from build123d import *

# Parameters (mm, degrees)
ESBO_O1_R                                      = 4.7625
RESSALTO_EXTRUS_O1_DEPTH                       = 151.9
FURO_ROSCADO_DE_M5X0_81_D                      = 4.2
FURO_ROSCADO_DE_M5X0_81_DEPTH                  = 14
FURO_ROSCADO_DE_M5X0_81_TIP                    = 1.2618073
FILETE1_R                                      = 0.5
BROCA_DE_ROSQUEAR_PARA_TARRAXA_DE_M3X0_5_D     = 2.5
BROCA_DE_ROSQUEAR_PARA_TARRAXA_DE_M3X0_5_DEPTH = 5
BROCA_DE_ROSQUEAR_PARA_TARRAXA_DE_M3X0_5_TIP   = 0.751075774
FILETE2_R                                      = 0.5
BROCA_DE_ROSQUEAR_PARA_TARRAXA_DE_M3_2_D       = 2.5
BROCA_DE_ROSQUEAR_PARA_TARRAXA_DE_M3_2_DEPTH   = 10
BROCA_DE_ROSQUEAR_PARA_TARRAXA_DE_M3_2_TIP     = 0.751075774


with BuildPart() as part:
    # Esboço1 → Ressalto-extrusão1 (new body)
    with BuildSketch(Plane.XY):
        with Locations((21.9, 0.462441068)):
            Circle(ESBO_O1_R)
    extrude(amount=RESSALTO_EXTRUS_O1_DEPTH)

    # Furo roscado de M5x0.81
    with Locations(Plane(origin=(0, 0, 0), x_dir=(-1, 0, 0), z_dir=(0, 0, -1))):
        with Locations((-21.9, 0.462441068)):
            Hole(FURO_ROSCADO_DE_M5X0_81_D / 2, depth=FURO_ROSCADO_DE_M5X0_81_DEPTH)
            with Locations((0, 0, -(FURO_ROSCADO_DE_M5X0_81_DEPTH + FURO_ROSCADO_DE_M5X0_81_TIP / 2))):  # 118° drill point
                Cone(0, FURO_ROSCADO_DE_M5X0_81_D / 2, FURO_ROSCADO_DE_M5X0_81_TIP, mode=Mode.SUBTRACT)

    # Filete1
    filete1_edges = [part.edges().sort_by_distance(p)[0] for p in [
        (17.1375, 0.462441068, 0),
    ]]
    fillet(filete1_edges, radius=FILETE1_R)

    # Broca de rosquear para tarraxa de M3x0.5
    with Locations(Plane.XY.offset(151.9)):
        with Locations((21.9, 0.462441068)):
            Hole(BROCA_DE_ROSQUEAR_PARA_TARRAXA_DE_M3X0_5_D / 2, depth=BROCA_DE_ROSQUEAR_PARA_TARRAXA_DE_M3X0_5_DEPTH)
            with Locations((0, 0, -(BROCA_DE_ROSQUEAR_PARA_TARRAXA_DE_M3X0_5_DEPTH + BROCA_DE_ROSQUEAR_PARA_TARRAXA_DE_M3X0_5_TIP / 2))):  # 118° drill point
                Cone(0, BROCA_DE_ROSQUEAR_PARA_TARRAXA_DE_M3X0_5_D / 2, BROCA_DE_ROSQUEAR_PARA_TARRAXA_DE_M3X0_5_TIP, mode=Mode.SUBTRACT)

    # Filete2
    filete2_edges = [part.edges().sort_by_distance(p)[0] for p in [
        (17.1375, 0.462441068, 151.9),
    ]]
    fillet(filete2_edges, radius=FILETE2_R)

    # Broca de rosquear para tarraxa de M3 2
    with Locations(Plane(origin=(18.970347391, -3.292361436, 26.879843119), x_dir=(-0.78840997447, 0.615150154154, 0), z_dir=(-0.615150154154, -0.78840997447, 0))):
        with Locations((0, 0)):
            Hole(BROCA_DE_ROSQUEAR_PARA_TARRAXA_DE_M3_2_D / 2, depth=BROCA_DE_ROSQUEAR_PARA_TARRAXA_DE_M3_2_DEPTH)
            with Locations((0, 0, -(BROCA_DE_ROSQUEAR_PARA_TARRAXA_DE_M3_2_DEPTH + BROCA_DE_ROSQUEAR_PARA_TARRAXA_DE_M3_2_TIP / 2))):  # 118° drill point
                Cone(0, BROCA_DE_ROSQUEAR_PARA_TARRAXA_DE_M3_2_D / 2, BROCA_DE_ROSQUEAR_PARA_TARRAXA_DE_M3_2_TIP, mode=Mode.SUBTRACT)


solid = part.part
Could you check a few things on this model? Use its own coordinates, in mm. A direction names the side the tool comes from. Coordinates: 2 decimals unless noted, no trailing zeros. Write each loop counter-clockwise with the first axis right and the second up, starting at its lowest first coordinate (ties: lowest second). Pieces come first, ordered by that corner, then holes. Notation, with made-up numbers: (-35.5, 16) - (-27.5, 16) arc R24 cw to (-27.5, 27) - close; hole circle Ø11 at (-34.5, 63). An arc over 180 degrees is marked (long way). Write item = value, one per line.
1) We'd pull the mould along X, two halves only. Please class faces 1 (the cylindrical face through (26.443, 1.893, 74.894)), 2 (the flat face through (20.9, 1.5, 151.9)), 3 (the cylindrical face through (21.73, 0.68, 28.1)): +X half, -X half, draft (parallel to the pull), parting line (faces both ways), or undercut.
Result set:
face_1 = parting line
face_2 = draft
face_3 = undercut
2) For faces 4 (the cylindrical face through (23.15, 0.52, 149.36)), 5 (the cylindrical face through (23.9, 1.1, 7.1)), 6 (the flat face through (19.9, 1.5, 0)), which set-ups out of +Z, -Z, +X, -X, +Y, -Y let a thin tool reach every point of the face, with its end or its side?
Result set:
face_4 = +Z
face_5 = -Z
face_6 = -Z, +X, -X, +Y, -Y
3) Please list where these lines run through material, in increasing order: line 1 (X direction, y = 0.5, z = 14); line 2 (Y direction, x = 21.9, z = 150.55); line 3 (X direction, y = 1.25, z = 12). Write a range as [from, to].
Result set:
line_1 = [17.14, 19.8], [24, 26.66]
line_2 = [-4.3, -0.79], [1.71, 5.22]
line_3 = [17.2, 19.95], [23.85, 26.6]
4) Will these pins go through, and if not, where does the flat tip stop? pin 1 Ø2.5 at (x, y) = (21.9, 0.46) entering from -Z; pin 2 Ø2 at (x, y) = (21.9, 0.46) entering from -Z.
Result set:
pin_1 = 14.51
pin_2 = 14.66
5) Suppose I cut it at A-A on z = 96. Please give me the cut outline in (x, y) (1 decimal), plus the area to 3 significant figures.
Result set:
outline = circle Ø9.5 at (21.9, 0.5)
area = 71.3 mm2
